Here's how the part is built. I have some questions about the finished solid (model axes, mm). Round coordinates to 2 decimals unless told otherwise and drop trailing zeros. Write each loop counter-clockwise with the first axis right and the second up, starting at its lowest first coordinate (ties: lowest second). Pieces come first, ordered by that corner, then holes. Notation, with made-up numbers: (10.5, 45) -> (57.5, 45) arc R25 cw to (57.5, 69) -> close; hole circle Ø2 at (31, 7). An arc over 180 degrees is marked (long way). Answer in a Markdown table with one row per item.
from build123d import *

# Parameters (mm, degrees)
SKETCH1_W           = 35
SKETCH1_H           = 10
BOSS_EXTRUDE1_DEPTH = 1
SKETCH2_R           = 0.25
SKETCH2_R_2         = 1.5
SKETCH2_W           = 0.4
SKETCH2_H           = 0.65
SKETCH2_W_2         = 0.3
SKETCH2_H_2         = 0.7
CUT_EXTRUDE1_DEPTH  = 1
SKETCH3_W           = 0.4
SKETCH3_H           = 0.65
BOSS_EXTRUDE2_DEPTH = 6


with BuildPart() as part:
    # Sketch1 → Boss-Extrude1 (new body)
    with BuildSketch(Plane(origin=(0, 0, 0), x_dir=(1, 0, 0), z_dir=(0, 1, 0))):
        Rectangle(SKETCH1_W, SKETCH1_H)
    extrude(amount=BOSS_EXTRUDE1_DEPTH)

    # Sketch2 → Cut-Extrude1 (cut)
    with BuildSketch(Plane.XZ):
        with Locations(Location((-9, 3.5, 0), (0, 0, 270))):
            Circle(SKETCH2_R)
        with Locations(Location((1.6, 3.5, 0), (0, 0, 270))):
            Circle(SKETCH2_R)
        with Locations(Location((-14.620013046, 0, 0), (0, 0, 270))):
            Circle(SKETCH2_R_2)
        with Locations((-9, 0)):
            Rectangle(SKETCH2_W, SKETCH2_H)
        with Locations((-9, -1.5)):
            Rectangle(SKETCH2_W, SKETCH2_H)
        with Locations((-5.3, 0)):
            Rectangle(SKETCH2_W, SKETCH2_H)
        with Locations((-5.3, -1.5)):
            Rectangle(SKETCH2_W, SKETCH2_H)
        with Locations((8, -0.325)):
            Rectangle(SKETCH2_W_2, SKETCH2_H_2)
        with Locations((3, 2.175)):
            Rectangle(SKETCH2_W_2, SKETCH2_H_2)
        with Locations((3, -2.825)):
            Rectangle(SKETCH2_W_2, SKETCH2_H_2)
    extrude(amount=-CUT_EXTRUDE1_DEPTH, mode=Mode.SUBTRACT)

    # Sketch3 → Boss-Extrude2 (add)
    with BuildSketch(Plane(origin=(0, 1, 0), x_dir=(1, 0, 0), z_dir=(0, 1, 0))):
        with Locations((10, -0.487564974)):
            Rectangle(SKETCH3_W, SKETCH3_H)
        with Locations((10, 3.512435026)):
            Rectangle(SKETCH3_W, SKETCH3_H)
        with Locations((10, -4.487564974)):
            Rectangle(SKETCH3_W, SKETCH3_H)
    extrude(amount=BOSS_EXTRUDE2_DEPTH)


solid = part.part
1) I want a section at C-C, the plane x = -3.5. List the corners of the cut face in (y, z) for me, and give its area (3 significant figures).
Response:
| item | result |
|---|---|
| outline | (0, -5) -> (1, -5) -> (1, 5) -> (0, 5) -> close |
| area | 10.0 mm^2 |
2) I want a section at B-B, the plane x = -13.5. List the corners of the cut face in (y, z) for me.
Response:
| item | result |
|---|---|
| outline | (0, -5) -> (1, -5) -> (1, -1) -> (0, -1) -> close; (0, 1) -> (1, 1) -> (1, 5) -> (0, 5) -> close |
3) We'd pull the mould along Z, two halves only. Please class faces 1 (the face through (-13.133, 0.493, 0.195)), 2 (the face through (17.5, 0.5, 0.1)), 3 (the face through (-0.2, 0.5, -5)): +Z half, -Z half, draft (parallel to the pull), parting line (faces both ways), or undercut.
Response:
| item | result |
|---|---|
| face 1 | undercut |
| face 2 | draft |
| face 3 | -Z half |
4) I want a section at A-A, the plane y = 3.5. List the corners of the cut face in (x, z) for me, and give its area (3 significant figures).
Response:
| item | result |
|---|---|
| outline | (9.8, -3.84) -> (10.2, -3.84) -> (10.2, -3.19) -> (9.8, -3.19) -> close; (9.8, 0.16) -> (10.2, 0.16) -> (10.2, 0.81) -> (9.8, 0.81) -> close; (9.8, 4.16) -> (10.2, 4.16) -> (10.2, 4.81) -> (9.8, 4.81) -> close |
| area | 0.780 mm^2 |
5) I need wall thicknesses on line 1 (X direction, y = 0.5, z = 3.5); line 2 (Y direction, x = 9.5, z = -0.5); line 3 (X direction, y = 6.75, z = 4.5). Which ranges of each line are inside material? Lowest first, please. Write a range as [from, to].
Response:
| item | result |
|---|---|
| line 1 | x = [-17.5, -9.25], [-8.75, 1.35], [1.85, 17.5] |
| line 2 | y = [0, 1] |
| line 3 | x = [9.8, 10.2] |
6) For pin 1 (5 mm diameter, centred on x = -6, z = 1.5, fed in from +Y); pin 2 (2.5 mm diameter, centred on x = -14.62, z = 0, fed in from +Y); pin 3 (0.7 mm diameter, centred on y = 3, z = -3.5, fed in from -X); pin 4 (0.7 mm diameter, centred on y = 2.5, z = 0.5, fed in from +X), each with a flat end and sliding along its axis, tell me the tip position at first contact or that it passes through.
Response:
| item | result |
|---|---|
| pin 1 | stops at y = 1 |
| pin 2 | passes through |
| pin 3 | stops at x = 9.8 |
| pin 4 | stops at x = 10.2 |
